The listing builds one solid part. Answer for the finished solid, in the listing's coordinates (mm). A direction names the side the tool comes from. Round coordinates to 2 decimals unless told otherwise and drop trailing zeros. Loops run counter-clockwise (first coordinate to the right, second up) from the corner with the lowest first, then second, coordinate; pieces in that order, holes last. Notation, with made-up numbers: (6, 42) -> (52, 42) arc R14 ccw to (52, 67) -> close; hole circle Ø2 at (-24, 60). An arc over 180 degrees is marked (long way). Use a Markdown table: item, result. Add a question column.
Q1. Section D-D on z = 37.5 is taken. Give the vertices of the cut face in (x, y), then the cut area to 3 significant figures.
Q2. Given pin 1 Ø5 at (x, y) = (-4, -0.5) entering from +Z; pin 2 Ø2.5 at (x, z) = (0, 5) entering from -Y, each flat-ended and moving along its own axis, determine where each tip first touches the part or whether it passes through.
Q3. Section A-A on z = 5 is taken. Give the vertices of the cut face in (x, y), then the cut area to 3 significant figures.
Q4. For a pull along Z with two mould halves and no side action, classify faces 1 (the cylindrical face through (0.07, 6.76, 23.5)), 2 (the flat face through (7.5, 0, 49)), 3 (the cylindrical face through (-0.575, -6.74, 6.386)), 4 (the flat face through (-7, 0, 0)) as released by +Z, released by -Z, zero draft, split by the parting line, or undercut.
Q5. Section B-B on y = -3.5 is taken. Give the vertices of the cut face in (x, z), then the cut area to 3 significant figures.
Q6. Which of the six approach directions +Z, -Z, +X, -X, +Y, -Y give full straight-line access (tool end or side, diameter ignored) to faces 5 (the flat face through (0, -6, 51)), 6 (the cylindrical face through (-0.575, 6.76, 6.386))?
Q7. Consider line 1 (X direction, y = -5.75, z = 59); line 2 (X direction, y = 6.8, z = 5). Determine where each line is inside the solid, lowest interval first.
from build123d import *

# Parameters (mm, degrees)
ESQUISSE1_W                = 15
ESQUISSE1_H                = 15
EXTRUSION1_DEPTH           = 100
ESQUISSE2_W                = 12
ESQUISSE2_H                = 12
EXTRUSION2_DEPTH           = 101.560926806
ESQUISSE3_R                = 1.5
EXTRUSION3_DEPTH           = 102.396498953
R_P_TITION_LIN_AIRE1_COUNT = 2
R_P_TITION_LIN_AIRE1_PITCH = 20


with BuildPart() as part:
    # Esquisse1 → Extrusion1 (new body)
    with BuildSketch(Plane.XY):
        Rectangle(ESQUISSE1_W, ESQUISSE1_H)
    extrude(amount=EXTRUSION1_DEPTH)

    # Esquisse2 → Extrusion2 (cut, through all)
    with BuildSketch(Plane.XY.offset(100)):
        Rectangle(ESQUISSE2_W, ESQUISSE2_H)
    extrude(amount=-EXTRUSION2_DEPTH, mode=Mode.SUBTRACT)

    # Esquisse3 → Extrusion3 (cut, through all)
    with BuildSketch(Plane(origin=(0, 7.5, 0), x_dir=(1, 0, 0), z_dir=(0, 1, 0))):
        with Locations(Location((0, -5, 0), (0, 0, 270))):
            Circle(ESQUISSE3_R)
    extrusion3 = extrude(amount=-EXTRUSION3_DEPTH, mode=Mode.SUBTRACT)

    # Répétition linéaire1: Extrusion3 ×2
    with Locations(*[(0, 0, i * R_P_TITION_LIN_AIRE1_PITCH) for i in range(1, R_P_TITION_LIN_AIRE1_COUNT)]):
        add(extrusion3, mode=Mode.SUBTRACT)


solid = part.part
Checked values:
| question | item | result |
|---|---|---|
| 1 | outline | (-7.5, -7.5) -> (7.5, -7.5) -> (7.5, 7.5) -> (-7.5, 7.5) -> close; hole (-6, -6) -> (6, -6) -> (6, 6) -> (-6, 6) -> close |
| 1 | area | 81.0 mm2 |
| 2 | pin 1 | stops at z = 100 |
| 2 | pin 2 | passes through |
| 3 | outline | (-7.5, -7.5) -> (-1.5, -7.5) -> (-1.5, -6) -> (-6, -6) -> (-6, 6) -> (-1.5, 6) -> (-1.5, 7.5) -> (-7.5, 7.5) -> close; (1.5, -7.5) -> (7.5, -7.5) -> (7.5, 7.5) -> (1.5, 7.5) -> (1.5, 6) -> (6, 6) -> (6, -6) -> (1.5, -6) -> close |
| 3 | area | 72.0 mm2 |
| 4 | face 1 | undercut |
| 4 | face 2 | zero draft |
| 4 | face 3 | undercut |
| 4 | face 4 | released by -Z |
| 5 | outline | (-7.5, 0) -> (-6, 0) -> (-6, 100) -> (-7.5, 100) -> close; (6, 0) -> (7.5, 0) -> (7.5, 100) -> (6, 100) -> close |
| 5 | area | 300 mm2 |
| 6 | face 5 | +Z, -Z |
| 6 | face 6 | +Y, -Y |
| 7 | line 1 | x = -7.5 to -6, 6 to 7.5 |
| 7 | line 2 | x = -7.5 to -1.5, 1.5 to 7.5 |
